```python
from build123d import *

# Parameters (mm, degrees)
F0_R     = 50.782965
F1_DEPTH = 500
F4_R     = 30.052271
F5_DEPTH = 37


with BuildPart() as f1:
    # F0 (on Top) → F1 (new body)
    with BuildSketch(Plane.XY):
        Circle(F0_R)
    extrude(amount=F1_DEPTH)

    # F2 (on Front) → F3 (revolve)
    with BuildSketch(Plane.XZ):
        Polygon((93.926854, 500), (0, 542.704165), (0, 500), align=None)
    revolve(axis=Axis((0, 0, 521.352082), (0, 0, -1)))

    # F4 (on face) → F5 (join)
    with BuildSketch(Plane(origin=(0, 0, 0), x_dir=(1, 0, 0), z_dir=(0, 0, -1))):
        Circle(F4_R)
    extrude(amount=F5_DEPTH)


solid = f1.part
```
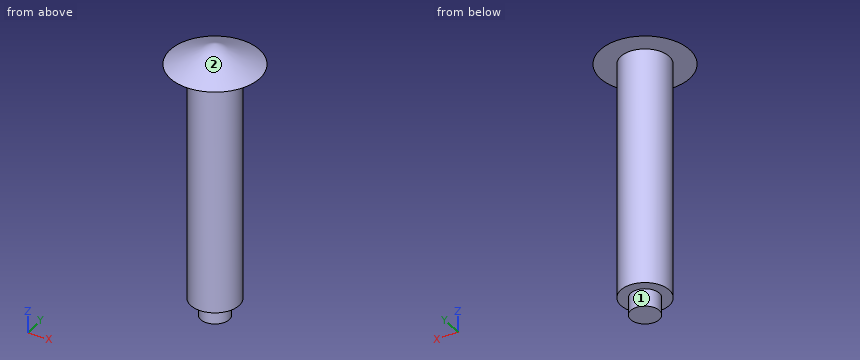
Could you check a few things on this model? Use its own coordinates, in mm. Face numbers are marked on the shaded views. A direction names the side the tool comes from. Round coordinates to 2 decimals unless told otherwise and drop trailing zeros. Loops run counter-clockwise (first coordinate to the right, second up) from the corner with the lowest first, then second, coordinate; pieces in that order, holes last. Notation, with made-up numbers: (19.5, 53.25) - (53.5, 53.25) arc R30 cw to (53.5, 79.25) - close; hole circle Ø4 at (65, -12.5). An arc over 180 degrees is marked (long way). Answer in a Markdown table with one row per item. Add a question column.
(1) I need wall thicknesses on line 1 along Y through (x, z) = (-41, 413.5); line 2 along Z through (x, y) = (51.5, -20.5); line 3 along Z through (x, y) = (-9, -15). Which ranges of each line are inside material? Lowest first, please.
(2) I'm going to push flat-ended pins straight in: pin 1 (8 mm diameter, centred on x = 2, y = 74, fed in from +Z); pin 2 (12 mm diameter, centred on x = 31.5, y = -24, fed in from -Z); pin 3 (10 mm diameter, centred on x = 36, y = -58.5, fed in from -Z). Where does each tip first touch, or does it pass through?
(3) For the marked faces 1 and 2, which set-ups out of +Z, -Z, +X, -X, +Y, -Y let a thin tool reach every point of the face, with its end or its side?
(4) If we section it at A-A (z = 136): Please give me the cut outline in (x, y).
Model answer:
| question | item | result |
|---|---|---|
| 1 | line 1 | y = -29.97 to 29.97 |
| 1 | line 2 | z = 500 to 517.5 |
| 1 | line 3 | z = -37 to 534.75 |
| 2 | pin 1 | stops at z = 510.87 |
| 2 | pin 2 | stops at z = 0 |
| 2 | pin 3 | stops at z = 500 |
| 3 | face 1 | -Z |
| 3 | face 2 | +Z |
| 4 | outline | circle Ø101.57 at (0, 0) |
